The model under review builds one solid part; all positions refer to its coordinate system, in mm. Coordinates: 2 decimals unless noted, no trailing zeros. Write each loop counter-clockwise with the first axis right and the second up, starting at its lowest first coordinate (ties: lowest second). Pieces come first, ordered by that corner, then holes. Notation, with made-up numbers: (19.5, -23.75) - (48.5, -23.75) arc R27 cw to (48.5, 2.25) - close; hole circle Ø6 at (50, -31.5). An arc over 180 degrees is marked (long way). Put each result on its own line as item: value.
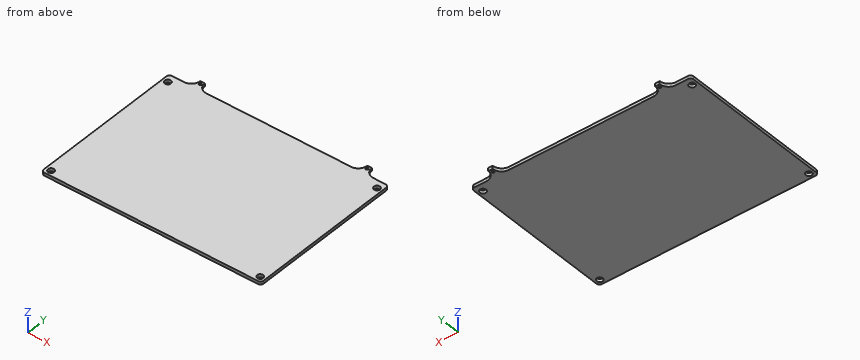
Autodesk Inventor part; units mm, degrees
ref_plane "YZ Plane" through (0, 0, 0) normal (1, 0, 0) x (0, 1, 0)
ref_plane "XZ Plane" through (0, 0, 0) normal (0, 1, 0) x (-1, 0, 0)
ref_plane "XY Plane" through (0, 0, 0) normal (0, 0, 1) x (1, 0, 0)
sketch "Sketch1" plane through (0, 0, 0) normal (0, 0, 1) x (1, 0, 0)
  ellipse E0 centre (-218.5917, 142.4744) end of major axis (-220.586, 142.4744) minor radius 1.993
  ellipse E1 centre (55.7593, 142.4744) end of major axis (53.765, 142.4744) minor radius 1.993
  line L0 (-222.6278, 147.4744) -> (-215.1278, 147.4744)
  line L1 (52.1593, 147.4744) -> (59.6593, 147.4744)
  line L2 (99.1593, 127.7477) -> (99.1593, -118.8668)
  line L3 (-262.1278, 127.7477) -> (-262.1278, -118.8668)
  line L4 (-257.1278, -123.8668) -> (94.1593, -123.8668)
  line L5 (94.1593, 132.7477) -> (74.1593, 132.7477)
  line L6 (59.6593, 147.2477) -> (59.6593, 147.4744)
  line L7 (52.1593, 147.4744) -> (52.1593, 147.2477)
  line L8 (-215.1278, 147.2477) -> (-215.1278, 147.4744)
  line L9 (-222.6278, 147.4744) -> (-222.6278, 147.2477)
  line L10 (-237.1278, 132.7477) -> (-257.1278, 132.7477)
  arc A0 (59.6593, 147.2477) -> (74.1593, 132.7477) centre (74.1593, 147.2477) ccw
  arc A1 (37.6593, 132.7477) -> (52.1593, 147.2477) centre (37.6593, 147.2477) ccw
  arc A2 (-215.1278, 147.2477) -> (-200.6278, 132.7477) centre (-200.6278, 147.2477) ccw
  arc A3 (-237.1278, 132.7477) -> (-222.6278, 147.2477) centre (-237.1278, 147.2477) ccw
  line L11 (37.6593, 132.7477) -> (-200.6278, 132.7477)
  arc A4 (94.1593, -123.8668) -> (99.1593, -118.8668) centre (94.1593, -118.8668) ccw
  arc A5 (-262.1278, -118.8668) -> (-257.1278, -123.8668) centre (-257.1278, -118.8668) ccw
  arc A6 (-257.1278, 132.7477) -> (-262.1278, 127.7477) centre (-257.1278, 127.7477) ccw
  arc A7 (99.1593, 127.7477) -> (94.1593, 132.7477) centre (94.1593, 127.7477) ccw
  circle A8 centre (90.6553, 119.8422) radius 5
  circle A9 centre (90.6553, -115.1578) radius 5
  circle A10 centre (-253.3447, -115.1578) radius 5
  circle A11 centre (-253.3447, 119.8422) radius 5
  point P0 (-262.1278, -108.8668)
  point P1 (-247.1278, -123.8668)
  point P2 (-262.1278, 112.7477)
  point P3 (99.1593, 112.7477)
  point P4 (59.6593, 132.7477)
  point P5 (-222.6278, 132.7477)
  point P6 (-242.1278, 132.7477)
  point P7 (79.1593, 132.7477)
  point P8 (59.6593, 147.361)
  point P9 (84.1593, -123.8668)
  point P10 (99.1593, -108.8668)
  dimension "d3" = 7.5
  dimension "d4" = 7.5
  dimension "d18" = 5
  dimension "d28" = 14.7267
  dimension "d29" = 14.5
  dimension "d33" = 5
  dimension "d34" = 4.7733
  dimension "d36" = 5
  dimension "d37" = 5
  dimension "d39" = 5
extrude "Extrusion1" add sketch "Sketch1" along normal blind 5
properties part number "back plate" material "Nylon 6/6"
1. Consider section A-A on x = -92.5. State the section outline as (y, z) points, plus the area to 3 significant figures.
Determined:
outline: (-123.87, 0) - (132.75, 0) - (132.75, 5) - (-123.87, 5) - close
area: 1,280 mm^2
2. To check wall thickness, follow probe 1 along Y at (x, z) = (-78.5, 2); probe 2 along X at (y, z) = (118.5, 0.85); probe 3 along X at (y, z) = (117.5, 4.3). State the ranges of each line that lie inside material, in increasing order.
Determined:
probe 1: y = -123.87 to 132.75
probe 2: x = -262.13 to -258.16, -248.53 to 85.84, 95.47 to 99.16
probe 3: x = -262.13 to -257.76, -248.93 to 86.24, 95.07 to 99.16
3. Consider section B-B on z = 4.1. Give the number of separate pieces and of enclosed holes in the cut face, plus the area to 3 significant figures.
Determined:
separate pieces: 1
enclosed holes: 6
area: 92,800 mm^2
4. For pin 1 Ø6 at (x, y) = (90.66, -115.16) entering from -Z; pin 2 Ø1.5 at (x, z) = (-121, 3.5) entering from +Y, all flat-tipped, find the tip position at first contact; note any pin that passes through.
Determined:
pin 1: passes through
pin 2: stops at y = 132.75
